```python
from build123d import *

# Parameters (mm, degrees)
SKETCH1_W               = 381
SKETCH1_H               = 254
BASE_EXTRUDE_DEPTH      = 19.05
CUT_EXTRUDE1_DEPTH      = 20.05
CUT_EXTRUDE2_DEPTH      = 128
CUT_EXTRUDE2_DEPTH_BACK = 128
CHAMFER1_SIZE           = 9.525


with BuildPart() as part:
    # Sketch1 → Base-Extrude (new body)
    with BuildSketch(Plane(origin=(0, 0, 0), x_dir=(1, 0, 0), z_dir=(0, 1, 0))):
        Rectangle(SKETCH1_W, SKETCH1_H)
    extrude(amount=BASE_EXTRUDE_DEPTH)

    # Sketch2 → Boss-Revolve1 (revolve)
    with BuildSketch(Plane(origin=(0, 0, 0), x_dir=(0, 0, -1), z_dir=(1, 0, 0)), mode=Mode.PRIVATE) as boss_revolve1_sk:
        with BuildLine():
            Line((0, -31.75), (0, 0))
            Line((0, 0), (122.967221242, 0))
            ThreePointArc((122.967221242, 0), (63.5, -23.684442484), (0, -31.75))
        make_face()
    revolve(boss_revolve1_sk.sketch.rotate(Axis((0, -41.201658399, 0), (0, 1, 0)), 180), axis=Axis((0, -41.201658399, 0), (0, 1, 0)))  # turned: the seam where the file's is

    # Sketch4 → Cut-Extrude1 (cut, through all)
    with BuildSketch(Plane.XZ):
        with BuildLine():
            Line((-190.5, 53.975), (-165.1, 53.975))
            ThreePointArc((-165.1, 53.975), (-142.875, 76.2), (-165.1, 98.425))
            Line((-165.1, 98.425), (-190.5, 98.425))
            Line((-190.5, 98.425), (-190.5, 53.975))
        make_face()
        with BuildLine():
            Line((-190.5, -98.425), (-165.1, -98.425))
            ThreePointArc((-165.1, -98.425), (-142.875, -76.2), (-165.1, -53.975))
            Line((-165.1, -53.975), (-190.5, -53.975))
            Line((-190.5, -53.975), (-190.5, -98.425))
        make_face()
        with BuildLine():
            Line((190.5, -98.425), (165.1, -98.425))
            ThreePointArc((165.1, -98.425), (142.875, -76.2), (165.1, -53.975))
            Line((165.1, -53.975), (190.5, -53.975))
            Line((190.5, -53.975), (190.5, -98.425))
        make_face()
        with BuildLine():
            Line((165.1, 53.975), (190.5, 53.975))
            Line((190.5, 53.975), (190.5, 98.425))
            Line((190.5, 98.425), (165.1, 98.425))
            ThreePointArc((165.1, 98.425), (142.875, 76.2), (165.1, 53.975))
        make_face()
    extrude(amount=-CUT_EXTRUDE1_DEPTH, mode=Mode.SUBTRACT)

    # Sketch5 → Cut-Extrude2 (cut, two sides)
    with BuildSketch(Plane.XY) as cut_extrude2_sk:
        with BuildLine():
            Line((56.44003455, -25.4), (-56.44003455, -25.4))
            ThreePointArc((-56.44003455, -25.4), (0, -31.75), (56.44003455, -25.4))
        make_face()
    extrude(amount=CUT_EXTRUDE2_DEPTH, mode=Mode.SUBTRACT)
    extrude(cut_extrude2_sk.sketch, amount=-CUT_EXTRUDE2_DEPTH_BACK, mode=Mode.SUBTRACT)

    # Chamfer1
    chamfer1_edges = [part.edges().sort_by_distance(p)[0] for p in [
        (-190.5, 9.525, 127),
        (190.5, 9.525, 127),
        (190.5, 9.525, -127),
        (-190.5, 9.525, -127),
    ]]
    chamfer(chamfer1_edges, length=CHAMFER1_SIZE)


solid = part.part
```
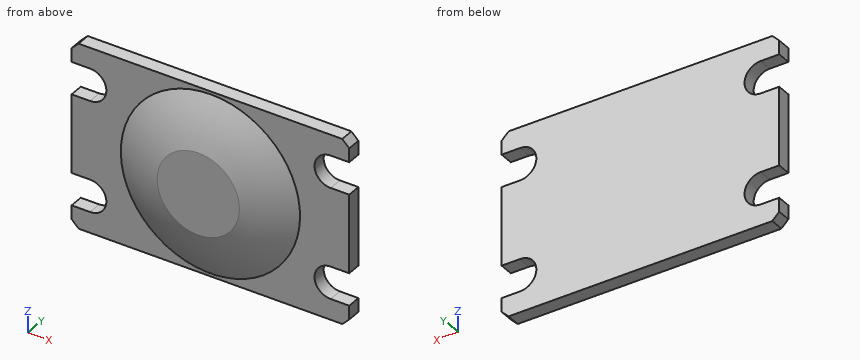
The listing builds one solid part. Answer for the finished solid, in the listing's coordinates (mm). Coordinates: 2 decimals unless noted, no trailing zeros. Write each loop counter-clockwise with the first axis right and the second up, starting at its lowest first coordinate (ties: lowest second). Pieces come first, ordered by that corner, then holes. Notation, with made-up numbers: (-10, -22.5) - (-1, -22.5) arc R21 ccw to (-1, 12.5) - close; hole circle Ø3 at (45, 81). An arc over 180 degrees is marked (long way). One line per item, written item: value.
1) Consider line 1 along Y through (x, z) = (145.5, -93); line 2 along X through (y, z) = (-2, 20.5); line 3 along Y through (x, z) = (-59.5, -37.5). Determine where each line is inside the solid, lowest interval first. Write a range as from..to.
Geometry check:
line 1: y = 0..19.05
line 2: x = -117.51..117.51
line 3: y = -21.82..19.05
2) Each of these flat-tipped pins is pushed along its axis until it touches: pin 1 Ø21 at (x, y) = (182, 6) entering from -Z; pin 2 Ø10 at (x, z) = (58.5, 68.5) entering from -Y; pin 3 Ø4 at (y, z) = (-4.5, -20) entering from +X; pin 4 Ø6 at (y, z) = (0.5, -65) entering from -X. Where does it stop, or does it pass through?
Geometry check:
pin 1: stops at z = -127
pin 2: stops at y = -17.08
pin 3: stops at x = 116.65
pin 4: stops at x = -148
3) Find section D-D (x = 21). Give the vertices of the cut face in (y, z), and give its area (3 significant figures).
Geometry check:
outline: (-25.4, -52.39) arc R253.13 ccw to (0, -121.16) - (0, -127) - (19.05, -127) - (19.05, 127) - (0, 127) - (0, 121.16) arc R253.13 ccw to (-25.4, 52.39) - close
area: 9,510 mm2
4) Find section C-C (z = 76.2). Give the vertices of the cut face in (x, y) (3 decimals).
Geometry check:
outline: (-142.875, 0) - (-96.512, 0) arc R242.301 ccw to (96.512, 0) - (142.875, 0) - (142.875, 19.05) - (-142.875, 19.05) - close
5) Find section A-A (y = 8). Give the vertices of the cut face in (x, z) (3 decimals).
Geometry check:
outline: (-190.5, -117.475) - (-180.975, -127) - (180.975, -127) - (190.5, -117.475) - (190.5, -98.425) - (165.1, -98.425) arc R22.225 cw to (165.1, -53.975) - (190.5, -53.975) - (190.5, 53.975) - (165.1, 53.975) arc R22.225 cw to (165.1, 98.425) - (190.5, 98.425) - (190.5, 117.475) - (180.975, 127) - (-180.975, 127) - (-190.5, 117.475) - (-190.5, 98.425) - (-165.1, 98.425) arc R22.225 cw to (-165.1, 53.975) - (-190.5, 53.975) - (-190.5, -53.975) - (-165.1, -53.975) arc R22.225 cw to (-165.1, -98.425) - (-190.5, -98.425) - close
6) Find section B-B (x = -42). Give the vertices of the cut face in (y, z).
Geometry check:
outline: (-25.4, -37.7) arc R250.5 ccw to (0, -115.57) - (0, -127) - (19.05, -127) - (19.05, 127) - (0, 127) - (0, 115.57) arc R250.5 ccw to (-25.4, 37.7) - close
